from build123d import *

# Parameters (mm, degrees)
F0_W     = 50.8
F0_H     = 38.1
F1_DEPTH = 6.35
F2_W     = 12.7
F2_H     = 12.7
F3_DEPTH = 12.701
F4_W     = 50.8
F4_H     = 19.05
F5_DEPTH = 50.8
F7_DEPTH = 19.051
F6_R     = 12.7
F8_DEPTH = 19.051


# Not quite as in the source:
# - a feature names something its author has since deleted; it is built from what else it names


with BuildPart() as f1:
    # F0 (on Top) → F1 (new body, symmetric)
    with BuildSketch(Plane.XY):
        Rectangle(F0_W, F0_H)
    extrude(amount=F1_DEPTH, both=True)

    # F2 (on face) → F3 (cut, through all)
    with BuildSketch(Plane.XY.offset(6.35)):
        with Locations((-19.05, 12.7)):
            Rectangle(F2_W, F2_H)
    extrude(amount=-F3_DEPTH, mode=Mode.SUBTRACT)

    # F4 (on face) → F5 (join)
    with BuildSketch(Plane.XY.offset(6.35)):
        with Locations((0, -9.525)):
            Rectangle(F4_W, F4_H)
    extrude(amount=F5_DEPTH)

    # F6 (on face) → F7 (cut, through all)
    with BuildSketch(Plane(origin=(0, 0, 0), x_dir=(-1, 0, 0), z_dir=(0, 1, 0))):
        with BuildLine():
            ThreePointArc((-25.4, 31.75), (-17.9605122618, 49.7105122225), (-5.57e-08, 57.15))
            Line((-5.57e-08, 57.15), (-25.4, 57.15))
            Line((-25.4, 57.15), (-25.4, 31.75))
        make_face()
        with BuildLine():
            ThreePointArc((-5.57e-08, 57.15), (17.9605122225, 49.7105122618), (25.4, 31.75))
            Line((25.4, 31.75), (25.4, 57.15))
            Line((25.4, 57.15), (-5.57e-08, 57.15))
        make_face()
    extrude(amount=-F7_DEPTH, mode=Mode.SUBTRACT)

    # F6 (on face) → F8 (cut, through all)
    with BuildSketch(Plane(origin=(0, 0, 0), x_dir=(-1, 0, 0), z_dir=(0, 1, 0))):
        with Locations((0, 31.75)):
            Circle(F6_R)
    extrude(amount=-F8_DEPTH, mode=Mode.SUBTRACT)


solid = f1.part
Read the model definition and answer for the solid it produces. Units are mm, in the model's axes. A direction names the side the tool comes from. Give positions to 0.01 mm unless a question says otherwise; leave off trailing zeros. Write each loop counter-clockwise with the first axis right and the second up, starting at its lowest first coordinate (ties: lowest second). Pieces come first, ordered by that corner, then holes. Notation, with made-up numbers: (26.25, 27) - (44.25, 27) arc R20 ccw to (44.25, 34) - close; hole circle Ø10 at (-10.75, 47). An arc over 180 degrees is marked (long way). Answer in a Markdown table with one row per item. Add a question column.
Item 1: Flat-ended cylindrical pins translate along their axes: P1, Ø1.5, axis at x = 9.5, z = 9, coming from the +Y side; P2, Ø20.5, axis at x = 0, z = 31.75, coming from the -Y side; P3, Ø5.5, axis at x = -10, y = 10.5, coming from the +Z side; P4, Ø8, axis at x = 11.5, y = -11.5, coming from the +Z side. Find the tip coordinate at first contact, or state that the pin passes through.
Item 2: Section D-D, the plane x = -1 is taken. Write down the section's boundary in (y, z), and give its area (3 significant figures).
Item 3: Section C-C, the plane z = 0 is taken. Write down the section's boundary in (x, y), and give its area (3 significant figures).
Item 4: A tool of negligible diameter and unlimited length cuts with its end or side. For faces 4 (the face through (6, 19.05, 0)), 5 (the face through (5, 10, 6.35)), 6 (the face through (-12.7, 13, 0)), from which of +Z, -Z, +X, -X, +Y, -Y can it reach the whole face along a straight path? Write none if from no direction.
Item 5: Find the intervals of material crossed by L1, parallel to Z at x = 10, y = 17; L2, parallel to Y at x = 15.5, z = 35.5; L3, parallel to X at y = -13, z = 31, in increasing order.
Item 6: Section A-A, the plane y = -12 is taken. Write down the section's boundary in (x, z).
Item 7: Section B-B, the plane x = 5.5 is taken. Write down the section's boundary in (y, z), and give its area (3 significant figures).
Item 8: Determine the mould class of faces 1 (the face through (-19, 6.35, 0)), 2 (the face through (25.4, -5, 8)), 3 (the face through (2.75, -9.39, 19.35)) for opening direction X: pulls with the +X half, pulls with the -X half, needs draft (parallel to the pull), parting line crosses it, or undercut.
Recorded:
| question | item | result |
|---|---|---|
| 1 | P1 | stops at y = 0 |
| 1 | P2 | passes through |
| 1 | P3 | stops at z = 6.35 |
| 1 | P4 | stops at z = 56.02 |
| 2 | outline | (-19.05, -6.35) - (19.05, -6.35) - (19.05, 6.35) - (0, 6.35) - (0, 19.09) - (-19.05, 19.09) - close; (-19.05, 44.41) - (0, 44.41) - (0, 57.13) - (-19.05, 57.13) - close |
| 2 | area | 969 mm2 |
| 3 | outline | (-25.4, -19.05) - (25.4, -19.05) - (25.4, 19.05) - (-12.7, 19.05) - (-12.7, 6.35) - (-25.4, 6.35) - close |
| 3 | area | 1,770 mm2 |
| 4 | face 4 | +Z, -Z, +X, -X, +Y |
| 4 | face 5 | +Z, +X, -X, +Y |
| 4 | face 6 | +Z, -Z, -X, +Y |
| 5 | L1 | z = -6.35 to 6.35 |
| 5 | L2 | y = -19.05 to 0 |
| 5 | L3 | x = -25.4 to -12.68, 12.68 to 25.4 |
| 6 | outline | (-25.4, -6.35) - (25.4, -6.35) - (25.4, 31.75) arc R25.4 ccw to (-25.4, 31.75) - close; hole circle Ø25.4 at (0, 31.75) |
| 7 | outline | (-19.05, -6.35) - (19.05, -6.35) - (19.05, 6.35) - (0, 6.35) - (0, 20.3) - (-19.05, 20.3) - close; (-19.05, 43.2) - (0, 43.2) - (0, 56.55) - (-19.05, 56.55) - close |
| 7 | area | 1,000 mm2 |
| 8 | face 1 | needs draft |
| 8 | face 2 | pulls with the +X half |
| 8 | face 3 | undercut |
